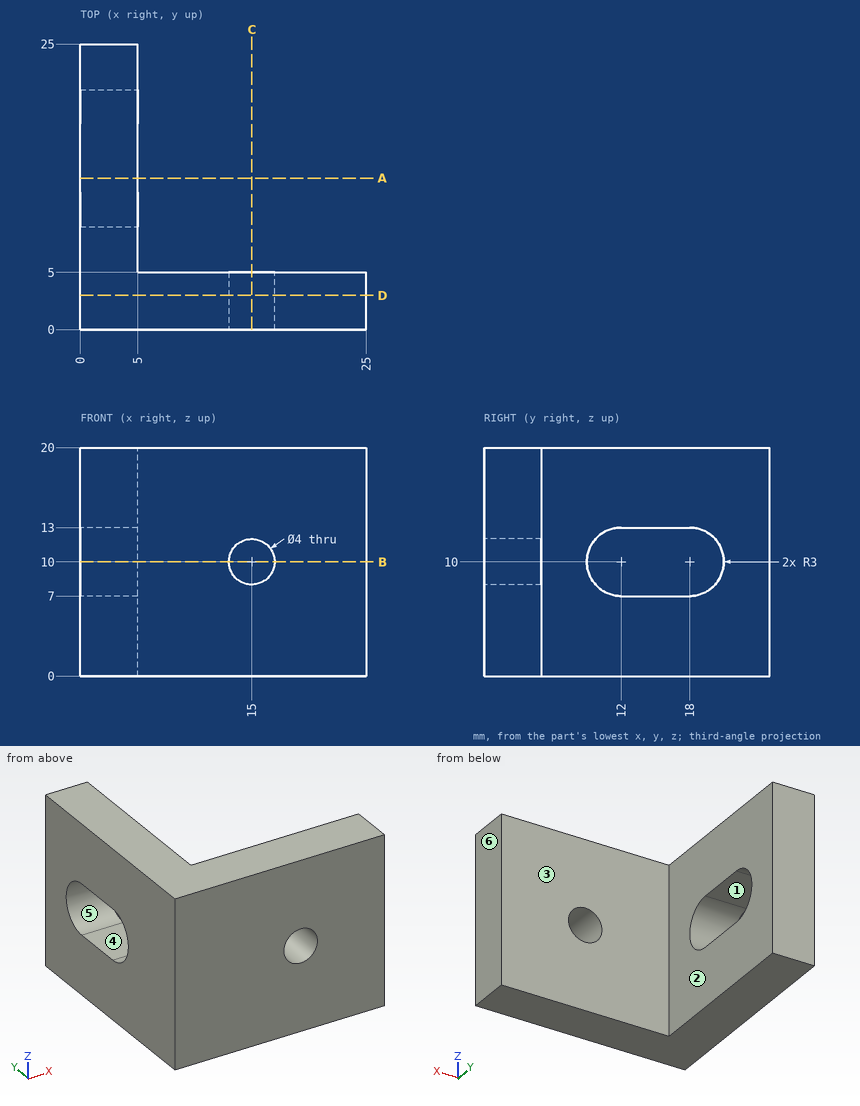
Geometry: see drawing. Coordinates: mm, zero at the bounding-box minimum. A direction names the side the tool comes from. Give positions to 0.01 mm unless a question says otherwise; leave off trailing zeros. Loops run counter-clockwise (first coordinate to the right, second up) from the corner with the lowest first, then second, coordinate; pieces in that order, holes last. Notation, with made-up numbers: (39.5, 42.5) -> (97.5, 42.5) arc R29 ccw to (97.5, 72.5) -> close; hole circle Ø6 at (30.5, 38). An arc over 180 degrees is marked (long way). Put each result on its own line as item: value.
1. Cut plane D-D (y = 3). Return the cut outline in (x, z), plus the area to 3 significant figures.
Taken from the geometry:
outline: (0, 0) -> (25, 0) -> (25, 20) -> (0, 20) -> close; hole circle Ø4 at (15, 10)
area: 487 mm2
2. Pull-direction query (Y, two-part tool) for the marked faces 1, 2, 3 and 4; classes: released by +Y, released by -Y, zero draft, split by the parting line, or undercut.
Taken from the geometry:
face 1: undercut
face 2: zero draft
face 3: released by +Y
face 4: undercut
3. Cut plane C-C (x = 15). Return the cut outline in (y, z).
Taken from the geometry:
outline: (0, 0) -> (5, 0) -> (5, 8) -> (0, 8) -> close; (0, 12) -> (5, 12) -> (5, 20) -> (0, 20) -> close
4. Ray query, line 1 along Z through (x, y) = (15, 2.9); line 2 along X through (y, z) = (3, 10); line 3 along Y through (x, z) = (13, 13.25). Return the intervals inside material, ascending. Write a range as [from, to].
Taken from the geometry:
line 1: z = [0, 8], [12, 20]
line 2: x = [0, 13], [17, 25]
line 3: y = [0, 5]
5. Cut plane A-A (y = 13.25). Return the cut outline in (x, z).
Taken from the geometry:
outline: (0, 0) -> (5, 0) -> (5, 7) -> (0, 7) -> close; (0, 13) -> (5, 13) -> (5, 20) -> (0, 20) -> close
6. Cut plane B-B (z = 10). Return the cut outline in (x, y).
Taken from the geometry:
outline: (0, 0) -> (13, 0) -> (13, 5) -> (5, 5) -> (5, 9) -> (0, 9) -> close; (0, 21) -> (5, 21) -> (5, 25) -> (0, 25) -> close; (17, 0) -> (25, 0) -> (25, 5) -> (17, 5) -> close
7. Pin query (flat end, axial travel): P1, Ø1, axis at x = 9, z = 8, coming from the -Y side; P2, Ø10, axis at y = 18, z = 10, coming from the +X side; P3, Ø10, axis at x = 10.5, z = 7.5, coming from the +Y side. Return the tip coordinate at first contact, or that it passes through.
Taken from the geometry:
P1: stops at y = 0
P2: stops at x = 5
P3: stops at y = 5
8. Set-up query: the marked faces 5 and 6. Return all of +Z, -Z, +X, -X, +Y, -Y with unobstructed straight access to the full face (end or side cutting, diameter ignored); none if empty.
Taken from the geometry:
face 5: +X, -X
face 6: +Z, -Z, +X, +Y, -Y
